```python
from build123d import *

# Parameters (mm, degrees)
SKETCH1_W        = 31
SKETCH1_H        = 6
SKETCH1_R        = 1.375
BASE_DEPTH       = 6
WIRE_GROVE_DEPTH = 18.670597047


with BuildPart() as part:
    # Sketch1 → Base (new body)
    with BuildSketch(Plane.XY):
        Rectangle(SKETCH1_W, SKETCH1_H)
        with Locations((-8.5, 0)):
            Circle(SKETCH1_R, mode=Mode.SUBTRACT)
        with Locations((8.5, 0)):
            Circle(SKETCH1_R, mode=Mode.SUBTRACT)
    extrude(amount=BASE_DEPTH)

    # Sketch2 → Wire Grove (cut, through all)
    with BuildSketch(Plane(origin=(0, 3, 0), x_dir=(1, 0, 0), z_dir=(0, 1, 0))):
        with BuildLine():
            Line((-1.9, 0), (1.9, 0))
            ThreePointArc((1.9, 0), (0, -1.9), (-1.9, 0))
        make_face()
    extrude(amount=-WIRE_GROVE_DEPTH, mode=Mode.SUBTRACT)


solid = part.part
```
Source: CAD feature listing. Evaluate the final solid. Frame: model axes, mm. Give positions to 0.01 mm unless a question says otherwise; leave off trailing zeros. Loops run counter-clockwise (first coordinate to the right, second up) from the corner with the lowest first, then second, coordinate; pieces in that order, holes last. Notation, with made-up numbers: M -28,-37 L -19,-37 A10 cw -19,-31 Z; hole C 62.25,10.25 d11. An arc over 180 degrees is marked long. Put each result on its own line as item: value.
Q1. Section C-C (y = 0.6). Return the cut outline in (x, z), and give its area (3 significant figures).
Response values:
outline: M -15.5,0 L -9.74,0 L -9.74,6 L -15.5,6 Z; M -7.26,0 L -1.9,0 A1.9 cw 1.9,0 L 7.26,0 L 7.26,6 L -7.26,6 Z; M 9.74,0 L 15.5,0 L 15.5,6 L 9.74,6 Z
area: 151 mm²
Q2. Section D-D (z = 3.7). Return the cut outline in (x, y) (3 decimals).
Response values:
outline: M -15.5,-3 L 15.5,-3 L 15.5,3 L -15.5,3 Z; hole C -8.5,0 d2.75; hole C 8.5,0 d2.75
Q3. Line query: probe 1 along X at (y, z) = (-0.85, 1.4); probe 2 along Y at (x, z) = (-8.5, 4.25) (3 decimals); probe 3 along X at (y, z) = (0.9, 3.2). Output: solid intervals per line, ascending. Write a range as [from, to].
Response values:
probe 1: x = [-15.5, -9.58], [-7.42, -1.28], [1.28, 7.42], [9.58, 15.5]
probe 2: y = [-3, -1.375], [1.375, 3]
probe 3: x = [-15.5, -9.54], [-7.46, 7.46], [9.54, 15.5]
Q4. Mould query, pull axis X, two halves, no side actions, for faces 1 (the flat face through (-15.5, 0, 3)), 2 (the cylindrical face through (0, 0, 1.9)), 3 (the flat face through (0, 3, 3)), 4 (the cylindrical face through (7.126, 0.06, 2.958)). Classes: released by +X, released by -X, zero draft, split by the parting line, or undercut.
Response values:
face 1: released by -X
face 2: undercut
face 3: zero draft
face 4: undercut
Q5. Section B-B (x = -8.5). Return the cut outline in (y, z) (3 decimals), and give its area (3 significant figures).
Response values:
outline: M -3,0 L -1.375,0 L -1.375,6 L -3,6 Z; M 1.375,0 L 3,0 L 3,6 L 1.375,6 Z
area: 19.5 mm²
Q6. Section A-A (z = 0.5). Return the cut outline in (x, y) (3 decimals), and give its area (3 significant figures).
Response values:
outline: M -15.5,-3 L -1.833,-3 L -1.833,3 L -15.5,3 Z; M 1.833,-3 L 15.5,-3 L 15.5,3 L 1.833,3 Z; hole C -8.5,0 d2.75; hole C 8.5,0 d2.75
area: 152 mm²
